Verification items for the finished model (mm, model axes). A direction names the side the tool comes from. Give positions to 0.01 mm unless a question says otherwise; leave off trailing zeros. Order: outer loops, then holes, each group sorted by start corner. A loop starts at its lowest first (then second) coordinate and runs counter-clockwise, first axis right, second up.
Autodesk Inventor part; units mm, degrees
ref_plane "YZ Plane" through (0, 0, 0) normal (1, 0, 0) x (0, 1, 0)
ref_plane "XZ Plane" through (0, 0, 0) normal (0, 1, 0) x (-1, 0, 0)
ref_plane "XY Plane" through (0, 0, 0) normal (0, 0, 1) x (1, 0, 0)
sketch "Skizze1" plane through (0, 0, 0) normal (0, 0, 1) x (1, 0, 0)
  line L0 (12.8939, 18.6723) -> (2.8939, 18.6723)
  line L1 (2.8939, 18.6723) -> (2.8939, 15.6723)
  line L2 (2.8939, 15.6723) -> (12.8939, 15.6723)
  line L3 (12.8939, 15.6723) -> (12.8939, 18.6723)
  line L4 (12.8939, 9.0723) -> (2.8939, 9.0723)
  line L5 (2.8939, 9.0723) -> (2.8939, 6.0723)
  line L6 (2.8939, 6.0723) -> (12.8939, 6.0723)
  line L7 (12.8939, 6.0723) -> (12.8939, 9.0723)
  line L8 (12.8939, 15.6723) -> (12.8939, 12.3723) construction
  line L9 (12.8939, 12.3723) -> (12.8939, 9.0723) construction
  point P0 (0, 0)
  point P1 (7.8939, 9.0723)
  dimension "d0" = 10
  dimension "d1" = 3
  dimension "d2" = 3
  dimension "d3" = 6.6
extrude "Extrusion1" add sketch "Skizze1" along normal blind 20
fillet "Rundung1" radius 3 4 edges at (12.8939, 7.5723, 20) (12.8939, 17.1723, 20) (2.8939, 17.1723, 20) (2.8939, 7.5723, 20)
sketch "Skizze2" plane through (2.8939, 6.0723, 0) normal (0, -1, 0) x (1, 0, 0)
  circle A0 centre (5, 15) radius 5 construction
  line L0 (10, 0) -> (10, 17) construction
  line L1 (0, 0) -> (0, 17) construction
  line L2 (3, 20) -> (7, 20) construction
  point P0 (-2.8939, 0)
hole "Bohrung1" at (7.8939, 6.0723, 15) direction (0, 1, 0) diameter 3.242 end through all countersink diameter 9 countersink angle 90
sketch "Skizze3" plane through (2.8939, 15.6723, 0) normal (0, -1, 0) x (1, 0, 0)
  line L0 (0, 0) -> (10, 0)
  line L1 (10, 0) -> (10, 2)
  line L2 (10, 0) -> (10, 17)
  line L3 (10, 2) -> (0, 2)
  line L4 (0, 0) -> (0, 17)
  point P0 (-2.8939, 0)
  dimension "d15" = 2
extrude "Extrusion2" add sketch "Skizze3" along normal through all
sketch "Skizze4" plane through (2.8939, 15.6723, 2) normal (0, 0, 1) x (1, 0, 0)
  line L0 (10, -3.3) -> (10, 0) construction
  line L1 (10, -3.3) -> (10, -6.6) construction
  line L2 (0, -3.3) -> (0, -6.6) construction
  line L3 (0, 0) -> (0, -3.3) construction
  line L4 (7, 3) -> (3, 3) construction
  line L5 (0, 3) -> (0, 0) construction
  line L6 (-4, -3.3) -> (5, -3.3) construction
  line L7 (-4, -3.3) -> (4.9964, -3.0464) construction
  line L8 (-4, -3.3) -> (5, -3.3) construction
  line L9 (2.4974, -3.1169) -> (4.9964, -3.0464) construction
  line L10 (4.9964, -3.0464) -> (7.4954, -2.976) construction
  point P0 (-2.8939, -15.6723)
  dimension "d34" = 5
  dimension "d35" = 9
  dimension "d36" = 6.3
  dimension "d37" = 5
  dimension "d38" = 9
  dimension "d40" = 9
  dimension "d41" = -1.615
hole "Bohrung2" at (10.3893, 12.6964, 2) at (5.3913, 12.5555, 2) direction (0, 0, -1) diameter 2 end through all countersink diameter 5 countersink angle 90
sketch "Skizze5" plane through (2.8939, 6.0723, 0) normal (0, -1, 0) x (1, 0, 0)
  circle A0 centre (5, 15) radius 4.5
  point P0 (-2.8939, 0)
hole "Bohrung3" at (7.8939, 6.0723, 15) direction (0, 1, 0) diameter 4 depth 3
equation "\"d41\" = -schrägWinkel"
properties part number "HalterUmlenkrolleOVL" material "PC/ABS-Kunststoff, 3DDruck, PLA"
(1) Section check A-A, the plane z = 2.5. Enter the section's corners in (x, y).
Solved:
outline: (2.89, 6.07) - (12.89, 6.07) - (12.89, 9.07) - (2.89, 9.07) - close; (2.89, 15.67) - (12.89, 15.67) - (12.89, 18.67) - (2.89, 18.67) - close
(2) Set-up check for faces 1 (the flat face through (8, 17, 20)), 2 (the flat face through (8, 9.072, 11)): record each of +Z, -Z, +X, -X, +Y, -Y from which the full face is reachable in a straight line by a thin tool's end or side.
Solved:
face 1: +Z, +X, -X, +Y, -Y
face 2: +Z, +X, -X
(3) Section check B-B, the plane z = 15. Enter the section's corners in (x, y), then the cut area to 3 significant figures.
Solved:
outline: (2.89, 6.07) - (3.39, 6.07) - (5.89, 8.57) - (5.89, 9.07) - (2.89, 9.07) - close; (2.89, 15.67) - (6.27, 15.67) - (6.27, 18.67) - (2.89, 18.67) - close; (9.51, 15.67) - (12.89, 15.67) - (12.89, 18.67) - (9.51, 18.67) - close; (9.89, 8.57) - (12.39, 6.07) - (12.89, 6.07) - (12.89, 9.07) - (9.89, 9.07) - close
area: 32.0 mm2
(4) Section check C-C, the plane y = 16.75. Enter the section's corners in (x, z), then the cut area to 3 significant figures.
Solved:
outline: (2.89, 0) - (12.89, 0) - (12.89, 17) arc R3 ccw to (9.89, 20) - (5.89, 20) arc R3 ccw to (2.89, 17) - close; hole circle Ø3.24 at (7.89, 15)
area: 188 mm2
(5) Scan lines: line 1 (X direction, y = 17.35, z = 15); line 2 (Y direction, x = 4.5, z = 3.5); line 3 (Z direction, x = 4, y = 9.5). Record each from-to range of solid material in increasing order.
Solved:
line 1: x = 2.89 to 6.27, 9.51 to 12.89
line 2: y = 6.07 to 9.07, 15.67 to 18.67
line 3: z = 0 to 2
(6) Section check D-D, the plane x = 7.5. Give the number of separate pieces and of enclosed holes in the cut face, then the cut area to 3 significant figures.
Solved:
separate pieces: 3
enclosed holes: 0
area: 105 mm2
(7) Release check for a two-part mould opening along X. For faces 3 (the flat face through (8, 12, 0)), 4 (the cylindrical face through (5.1, 11.6, 0.2)), 5 (the flat face through (2.894, 8, 8)) record: pulls with the +X half, pulls with the -X half, needs draft (parallel to the pull), parting line crosses it, or undercut.
Solved:
face 3: needs draft
face 4: undercut
face 5: pulls with the -X half
(8) Go/stop test with flat-tipped pins: pin 1 (4 mm diameter, centred on x = 9, z = 16, fed in from -Y); pin 2 (3.5 mm diameter, centred on x = 6, y = 12.5, fed in from +Z); pin 3 (1.6 mm diameter, centred on x = 5.39, y = 12.56, fed in from -Z). Record where each tip stops, or that it passes through.
Solved:
pin 1: stops at y = 7.08
pin 2: stops at z = 1.86
pin 3: passes through
